Can you work these out from the model? Positions are in its coordinate system, mm. Give positions to 0.01 mm unless a question says otherwise; leave off trailing zeros. Loops run counter-clockwise (first coordinate to the right, second up) from the corner with the lowest first, then second, coordinate; pieces in that order, holes last. Notation, with made-up numbers: (9.5, 65) -> (57.5, 65) arc R27 ccw to (57.5, 98) -> close; hole circle Ø1 at (-21.5, 54). An arc over 180 degrees is marked (long way). Return JSON: item names as keys, results as strings. Group by question number.
Q1. Suppose I cut it at B-B, the plane z = -127.5. Please give me the cut outline in (x, y), and give its area (3 significant figures).
Q2. Will these pins go through, and if not, where does the flat tip stop? pin 1 (6.5 mm diameter, centred on x = 37, y = -15, fed in from -Z); pin 2 (3 mm diameter, centred on x = 14.5, z = -106.5, fed in from -Y); pin 3 (1.8 mm diameter, centred on x = 38.5, y = -31, fed in from +Z).
Q3. Suppose I cut it at A-A, the plane x = 20. Please give me the cut outline in (y, z).
Q4. I need wall thicknesses on line 1 along X through (y, z) = (-2.05, -126); line 2 along Y through (x, z) = (3.5, -129.5); line 3 along X through (y, z) = (-16.5, -42.5). Which ranges of each line are inside material? Lowest first, please. Write a range as [from, to].
Q5. Suppose I cut it at D-D, the plane z = -96.5. Please give me the cut outline in (x, y).
Q6. Suppose I cut it at C-C, the plane y = -33. Please give me the cut outline in (x, z).
```python
from build123d import *

# Parameters (mm, degrees)
BOSS_EXTRUDE1_DEPTH = 180
SKETCH2_W           = 23
SKETCH2_H           = 34
CUT_EXTRUDE1_DEPTH  = 200
SKETCH3_R           = 5
CUT_EXTRUDE2_DEPTH  = 200


with BuildPart() as part:
    # Sketch1 → Boss-Extrude1 (new body)
    with BuildSketch(Plane.XY):
        Polygon((0, 0), (40, 0), (40, -40), (34, -40), (34, -6), (0, -6), align=None)
    extrude(amount=-BOSS_EXTRUDE1_DEPTH)

    # Sketch2 → Cut-Extrude1 (cut)
    with BuildSketch(Plane.ZY.offset(-34)):
        with Locations((-11.5, -23)):
            Rectangle(SKETCH2_W, SKETCH2_H)
        with Locations((-168.5, -23)):
            Rectangle(SKETCH2_W, SKETCH2_H)
    extrude(amount=-CUT_EXTRUDE1_DEPTH, mode=Mode.SUBTRACT)

    # Sketch3 → Cut-Extrude2 (cut)
    with BuildSketch(Plane(origin=(0, 0, 0), x_dir=(1, 0, 0), z_dir=(0, 1, 0))):
        with Locations(Location((20, 126, 0), (0, 0, 270))):
            Circle(SKETCH3_R)
        with Locations(Location((20, 54, 0), (0, 0, 90))):
            Circle(SKETCH3_R)
    extrude(amount=-CUT_EXTRUDE2_DEPTH, mode=Mode.SUBTRACT)


solid = part.part
```
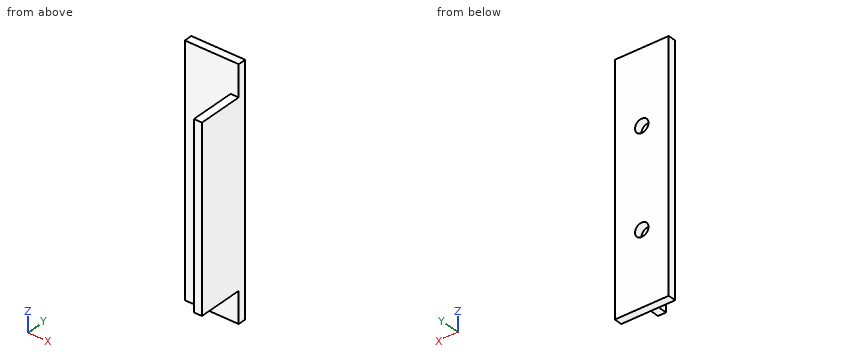
Ans:
{
 "1": {"outline": "(0, -6) -> (15.23, -6) -> (15.23, 0) -> (0, 0) -> close; (24.77, -6) -> (34, -6) -> (34, -40) -> (40, -40) -> (40, 0) -> (24.77, 0) -> close", "area": "387 mm^2"},
 "2": {"pin 1": "stops at z = -157", "pin 2": "stops at y = -6", "pin 3": "stops at z = -23"},
 "3": {"outline": "(-6, -180) -> (0, -180) -> (0, -131) -> (-6, -131) -> close; (-6, -121) -> (0, -121) -> (0, -59) -> (-6, -59) -> close; (-6, -49) -> (0, -49) -> (0, 0) -> (-6, 0) -> close"},
 "4": {"line 1": "x = [0, 15], [25, 40]", "line 2": "y = [-6, 0]", "line 3": "x = [34, 40]"},
 "5": {"outline": "(0, -6) -> (34, -6) -> (34, -40) -> (40, -40) -> (40, 0) -> (0, 0) -> close"},
 "6": {"outline": "(34, -157) -> (40, -157) -> (40, -23) -> (34, -23) -> close"}
}
